from build123d import *

# Parameters (mm, degrees)
SKETCH_1_R          = 21
EXTRUDE_1_DEPTH     = 3
EXTRUDE_START       = 9
SKETCH_2_R          = 21
EXTRUDE_2_DEPTH     = 9
SKETCH_3_R          = 1.6
CUT_EXTRUDE_1_DEPTH = 26.5
SKETCH_6_W          = 15
SKETCH_6_H          = 50
CUT_EXTRUDE_3_DEPTH = 7.5


with BuildPart() as part:
    # 草图1 → 凸台-拉伸1 (new body)
    with BuildSketch(Plane.XY):
        Circle(SKETCH_1_R)
    extrude(amount=EXTRUDE_1_DEPTH)

    # 草图2 → 凸台-拉伸2 (add)
    with BuildSketch(Plane(origin=(0, 0, 0), x_dir=(-1, 0, 0), z_dir=(0, 0, -1)).offset(EXTRUDE_START)):
        Circle(SKETCH_2_R)
    extrude(amount=-EXTRUDE_2_DEPTH)

    # 草图3 → 切除-拉伸1 (cut)
    with BuildSketch(Plane(origin=(0, 0, -9), x_dir=(-1, 0, 0), z_dir=(0, 0, -1))):
        with Locations((0, 13.5)):
            Circle(SKETCH_3_R)
        with Locations((11.691342951, -6.75)):
            Circle(SKETCH_3_R)
        with Locations((-11.691342951, -6.75)):
            Circle(SKETCH_3_R)
    extrude(amount=-CUT_EXTRUDE_1_DEPTH, mode=Mode.SUBTRACT)

    # 草图6 → 切除-拉伸3 (cut)
    with BuildSketch(Plane(origin=(0, 0, -9), x_dir=(-1, 0, 0), z_dir=(0, 0, -1))):
        Rectangle(SKETCH_6_W, SKETCH_6_H)
    extrude(amount=-CUT_EXTRUDE_3_DEPTH, mode=Mode.SUBTRACT)


solid = part.part
Build history of the part. All positions in model axes, mm. A direction names the side the tool comes from. Round coordinates to 2 decimals unless told otherwise and drop trailing zeros. Loops run counter-clockwise (first coordinate to the right, second up) from the corner with the lowest first, then second, coordinate; pieces in that order, holes last. Notation, with made-up numbers: (25, 11.5) -> (60, 11.5) arc R22 ccw to (60, 36.5) -> close; hole circle Ø2 at (-14.75, -32.75). An arc over 180 degrees is marked (long way). One line per item, written item: value. Start each with the question number.
Q1. Cut at A-A on z = -7. List the corners of the cut face in (x, y).
Q2. Cut at B-B on x = 0. List the corners of the cut face in (y, z).
Q3. Probe line 1 along X through (y, z) = (-7, -5); line 2 along X through (y, z) = (-13, -7.5); line 3 along Z through (x, y) = (3.5, 13.5). List the from-to ranges inside material, lowest first.
Q4. Cut at D-D on y = -6.75. List the corners of the cut face in (x, z), plus the area to 3 significant figures.
Q5. Drop flat-ended pins along their axis: pin 1 Ø1.9 at (x, y) = (11.69, -6.75) entering from -Z; pin 2 Ø1 at (y, z) = (1, 0) entering from -X; pin 3 Ø5 at (x, z) = (-5.5, -1) entering from -Y; pin 4 Ø6 at (y, z) = (9.5, -4.5) entering from +X. Give the stop position or say it passes through.
Q6. 3-axis set-ups, long thin cutter, end or side, ignore diameter. For faces 3 (the face through (7.5, 0, -5)), 4 (the face through (13, 0, -9)): which of +Z, -Z, +X, -X, +Y, -Y reach the whole face in a straight line?
Q7. Two-plate mould, pull along Y, no slides. Class faces 1 (the face through (-13, 0, -9)), 2 (the face through (10.95, -8.17, -3.08)): released by +Y, released by -Y, zero draft, split by the parting line, or undercut.
Q8. Cut at C-C on y = 13.5. List the corners of the cut face in (x, z).
Computed:
1. outline: (-7.5, -19.62) -> (-7.5, 19.62) arc R21 ccw to start; (7.5, -19.62) arc R21 ccw to (7.5, 19.62) -> close; hole circle Ø3.2 at (-11.69, -6.75); hole circle Ø3.2 at (11.69, -6.75)
2. outline: (-21, -1.5) -> (11.9, -1.5) -> (11.9, 3) -> (-21, 3) -> close; (15.1, -1.5) -> (21, -1.5) -> (21, 3) -> (15.1, 3) -> close
3. line 1: -19.8 to -13.27, -10.11 to -7.5, 7.5 to 10.11, 13.27 to 19.8
3. line 2: -16.49 to -7.5, 7.5 to 16.49
3. line 3: -1.5 to 3
4. outline: (-19.89, -9) -> (-13.29, -9) -> (-13.29, 3) -> (-19.89, 3) -> close; (-10.09, -9) -> (-7.5, -9) -> (-7.5, -1.5) -> (7.5, -1.5) -> (7.5, -9) -> (10.09, -9) -> (10.09, 3) -> (-10.09, 3) -> close; (13.29, -9) -> (19.89, -9) -> (19.89, 3) -> (13.29, 3) -> close
4. area: 288 mm²
5. pin 1: through
5. pin 2: x = -20.99
5. pin 3: y = -20.78
5. pin 4: x = 19.97
6. face 3: -Z, +Y, -Y
6. face 4: -Z, +X, -X, +Y, -Y
7. face 1: zero draft
7. face 2: undercut
8. outline: (-16.09, -9) -> (-7.5, -9) -> (-7.5, -1.5) -> (-1.6, -1.5) -> (-1.6, 3) -> (-16.09, 3) -> close; (1.6, -1.5) -> (7.5, -1.5) -> (7.5, -9) -> (16.09, -9) -> (16.09, 3) -> (1.6, 3) -> close
